Check sheet for the modelled part. Datum: model origin and axes. Units: mm. Give positions to 0.01 mm unless a question says otherwise; leave off trailing zeros. Order: outer loops, then holes, each group sorted by start corner. A loop starts at its lowest first (then second) coordinate and runs counter-clockwise, first axis right, second up.
Item 1: Sectioned sample at A-A on z = 1.75. Count the separate pieces of the cut face and the enclosed holes in it, and give its area (3 significant figures).
Item 2: Material ranges on line 1 along Y through (x, z) = (-62, 2.5); line 2 along X through (y, z) = (-4.5, 4); line 3 along Y through (x, z) = (-105, 3.8), recorded low to high.
Item 3: Gauge pin test, flat ends, axial feed: P1, Ø10.5, axis at x = -160, y = 20, coming from the +Z side; P2, Ø4.5, axis at x = 134, y = 0, coming from the -Z side. Record the tip position at first contact, or that the pin passes through.
Item 4: Sectioned sample at B-B on y = -9.5. Record the boundary of the cut face in (x, z), and give its area (3 significant figures).
Item 5: Release check for a two-part mould opening along X. For faces 1 (the cylindrical face through (-156.9, -19.02, 3.04)), 2 (the flat face through (-3, 1, 6)), 3 (the cylindrical face through (175.5, 4.88, 3.04)), 4 (the flat face through (-180, -40, 3)) record: released by +X, released by -X, zero draft, split by the parting line, or undercut.
from build123d import *

# Parameters (mm, degrees)
SKETCH_1_W          = 400
SKETCH_1_H          = 100
EXTRUDE_1_DEPTH     = 6
SKETCH_2_R          = 5
SKETCH_2_R_2        = 3.25
SKETCH_2_R_3        = 16.25
SKETCH_2_R_4        = 2.5
CUT_EXTRUDE_2_DEPTH = 207.242575624
SKETCH_3_R          = 3
SKETCH_3_R_2        = 2
SKETCH_3_R_3        = 2.5
CUT_EXTRUDE_3_DEPTH = 207.242575624


with BuildPart() as part:
    # 草圖1 → 伸長1 (new body)
    with BuildSketch(Plane.XY):
        Rectangle(SKETCH_1_W, SKETCH_1_H)
    extrude(amount=EXTRUDE_1_DEPTH)

    # 草圖2 → 伸長2 (cut, through all)
    with BuildSketch(Plane.XY.offset(6)):
        with Locations((-160, 0)):
            Circle(SKETCH_2_R)
        with Locations((-160, 20)):
            Circle(SKETCH_2_R_2)
        with Locations((-160, -20)):
            Circle(SKETCH_2_R_2)
        with Locations((160, 0)):
            Circle(SKETCH_2_R_3)
        with Locations((160, 26)):
            Circle(SKETCH_2_R_4)
        with Locations((134, 0)):
            Circle(SKETCH_2_R_4)
        with Locations((186, 0)):
            Circle(SKETCH_2_R_4)
        with Locations((160, -26)):
            Circle(SKETCH_2_R_4)
        Polygon((-200, -30), (-160, -50), (-200, -50), align=None)
        Polygon((200, -50), (200, -30), (160, -50), align=None)
    extrude(amount=-CUT_EXTRUDE_2_DEPTH, mode=Mode.SUBTRACT)

    # 草圖3 → 伸長3 (cut, through all)
    with BuildSketch(Plane.XY.offset(6)):
        with Locations((-105, 5)):
            Circle(SKETCH_3_R)
        with Locations((-35, 5)):
            Circle(SKETCH_3_R)
        with Locations((35, 5)):
            Circle(SKETCH_3_R)
        with Locations((105, 5)):
            Circle(SKETCH_3_R)
        with Locations((-62, -20)):
            Circle(SKETCH_3_R_2)
        with Locations((0, -20)):
            Circle(SKETCH_3_R_2)
        with Locations((62, -20)):
            Circle(SKETCH_3_R_2)
        with Locations((-192, -20)):
            Circle(SKETCH_3_R_2)
        with Locations((127, -20)):
            Circle(SKETCH_3_R_2)
        with Locations((-127, -20)):
            Circle(SKETCH_3_R_2)
        with Locations((192, -20)):
            Circle(SKETCH_3_R_2)
        with Locations((-70, -40)):
            Circle(SKETCH_3_R_3)
        with Locations((0, -40)):
            Circle(SKETCH_3_R_3)
        with Locations((70, -40)):
            Circle(SKETCH_3_R_3)
    extrude(amount=-CUT_EXTRUDE_3_DEPTH, mode=Mode.SUBTRACT)


solid = part.part
Report:
1. separate pieces: 1
1. enclosed holes: 22
1. area: 37,900 mm2
2. line 1: y = -50 to -22, -18 to 50
2. line 2: x = -200 to -162.18, -157.82 to 144.39, 175.61 to 200
2. line 3: y = -50 to 2, 8 to 50
3. P1: stops at z = 6
3. P2: passes through
4. outline: (-200, 0) - (146.82, 0) - (146.82, 6) - (-200, 6) - close; (173.18, 0) - (200, 0) - (200, 6) - (173.18, 6) - close
4. area: 2,240 mm2
5. face 1: undercut
5. face 2: zero draft
5. face 3: undercut
5. face 4: released by -X
